Here's how the part is built. I have some questions about the finished solid (model axes, mm). A direction names the side the tool comes from. Round coordinates to 2 decimals unless told otherwise and drop trailing zeros. Loops run counter-clockwise (first coordinate to the right, second up) from the corner with the lowest first, then second, coordinate; pieces in that order, holes last. Notation, with made-up numbers: (-21.75, 0.25) - (8.25, 0.25) arc R24 cw to (8.25, 12.25) - close; hole circle Ø3 at (-23.5, 72.5). An arc over 180 degrees is marked (long way). Answer as a JSON object with one key per item and string values. Group by question number.
1) I want a section at A-A, the plane x = -8.05. Please give me the cut outline in (y, z), then the cut area to 3 significant figures.
2) If I drill on line 1 along Y through (x, z) = (0, 17.95); line 2 along Z through (x, y) = (14, 29); line 3 along X through (y, z) = (28, 18.5), over which ranges is the centre line in solid material (lowest first)? Write a range as [from, to].
3) I want a section at C-C, the plane z = 8.05. Please give me the cut outline in (x, y), then the cut area to 3 significant figures.
4) Which directions (+Z, -Z, +X, -X, +Y, -Y) give clear straight access to the entire face, cutting with the end or side of a thin tool? Please do faces 1 (the face through (0, 26, -17)), 2 (the face through (0.08, 26.25, -18.48)).
5) I want a section at B-B, the plane y = 28.05. Please give me the cut outline in (x, z), then the cut area to 3 significant figures.
6) I want a section at D-D, the plane x = 14. Please give me the cut outline in (y, z), then the cut area to 3 significant figures.
7) If we mould it in two halves opening along Y, with no side actions, what happens to faces 3 (the face through (0, 40, -19)), 4 (the face through (-7.45, 1.52, 5.3)), 5 (the face through (-6.265, 20.234, 18.479))? For each: pulls with the +Y half, pulls with the -Y half, needs draft (parallel to the pull), parting line crosses it, or undercut.
8) Will these pins go through, and if not, where does the flat tip stop? P1, Ø10, axis at x = 9, z = 5.5, coming from the +Y side; P2, Ø3, axis at x = -5.69, z = 5.69, coming from the +Y side.
from build123d import *

# Parameters (mm, degrees)
C_1U_DEPTH               = 20
SKETCH_8_R               = 3.95
SKETCH_8_R_2             = 1.8
CUT_EXTRUDE_696_DEPTH    = 5
PATTERN_CIRCULAR_A_COUNT = 2
PATTERN_CIRCULAR_A_ANGLE = 270
PATTERN_CIRCULAR_B_COUNT = 2
PATTERN_CIRCULAR_B_ANGLE = 90


with BuildPart() as part:
    # c型梁 → C型梁1u (new, symmetric)
    with BuildSketch(Plane(origin=(0, 0, 0), x_dir=(0, 0, -1), z_dir=(1, 0, 0))):
        Polygon((-20, 0), (20, 0), (20, 40), (17, 40), (17, 3), (-17, 3), (-17, 40), (-20, 40), align=None)
    extrude(amount=C_1U_DEPTH, both=True)

    # 8位安装孔 → Cut-Extrude 696 (cut, symmetric)
    with BuildSketch(Plane(origin=(0, 3, 0), x_dir=(1, 0, 0), z_dir=(0, 1, 0))):
        with Locations(Location((0, 0, 0), (0, 0, 270))):
            Circle(SKETCH_8_R)
        with Locations(Location((8.05, 0, 0), (0, 0, 270))):
            Circle(SKETCH_8_R_2)
        with Locations(Location((5.692209589, -5.692209589, 0), (0, 0, 270))):
            Circle(SKETCH_8_R_2)
        with Locations(Location((0, -8.05, 0), (0, 0, 270))):
            Circle(SKETCH_8_R_2)
        with Locations(Location((-5.692209589, -5.692209589, 0), (0, 0, 270))):
            Circle(SKETCH_8_R_2)
        with Locations(Location((-8.05, 0, 0), (0, 0, 270))):
            Circle(SKETCH_8_R_2)
        with Locations(Location((-5.692209589, 5.692209589, 0), (0, 0, 270))):
            Circle(SKETCH_8_R_2)
        with Locations(Location((0, 8.05, 0), (0, 0, 270))):
            Circle(SKETCH_8_R_2)
        with Locations(Location((5.692209589, 5.692209589, 0), (0, 0, 270))):
            Circle(SKETCH_8_R_2)
    cut_extrude_696 = extrude(amount=CUT_EXTRUDE_696_DEPTH, both=True, mode=Mode.SUBTRACT)

    # 安装孔A侧: Cut-Extrude 696 ×2 about axis
    pattern_circular_a_axis = Axis((20, 3, 17), (-1, 0, 0))
    for i in range(1, PATTERN_CIRCULAR_A_COUNT):
        add(cut_extrude_696.rotate(pattern_circular_a_axis, i * PATTERN_CIRCULAR_A_ANGLE / (PATTERN_CIRCULAR_A_COUNT - 1)), mode=Mode.SUBTRACT)

    # 安装孔B侧: Cut-Extrude 696 ×2 about axis
    pattern_circular_b_axis = Axis((20, 3, -17), (-1, 0, 0))
    for i in range(1, PATTERN_CIRCULAR_B_COUNT):
        add(cut_extrude_696.rotate(pattern_circular_b_axis, i * PATTERN_CIRCULAR_B_ANGLE / (PATTERN_CIRCULAR_B_COUNT - 1)), mode=Mode.SUBTRACT)


solid = part.part
Outcome:
{
 "1": {"outline": "(0, -20) - (18.2, -20) - (18.2, -17) - (3, -17) - (3, -1.8) - (0, -1.8) - close; (0, 1.8) - (3, 1.8) - (3, 17) - (18.2, 17) - (18.2, 20) - (0, 20) - close; (21.8, -20) - (40, -20) - (40, -17) - (21.8, -17) - close; (21.8, 17) - (40, 17) - (40, 20) - (21.8, 20) - close", "area": "310 mm^2"},
 "2": {"line 1": "[0, 10.15], [13.75, 16.05], [23.95, 26.25], [29.85, 40]", "line 2": "[-20, -17], [17, 20]", "line 3": "[-20, -1.8], [1.8, 20]"},
 "3": {"outline": "(-20, 0) - (-1.8, 0) - (-1.8, 3) - (-20, 3) - close; (1.8, 0) - (20, 0) - (20, 3) - (1.8, 3) - close", "area": "109 mm^2"},
 "4": {"face 1": "+X, -X, +Y", "face 2": "+Z, -Z"},
 "5": {"outline": "(-20, -20) - (-1.8, -20) - (-1.8, -17) - (-20, -17) - close; (-20, 17) - (-1.8, 17) - (-1.8, 20) - (-20, 20) - close; (1.8, -20) - (20, -20) - (20, -17) - (1.8, -17) - close; (1.8, 17) - (20, 17) - (20, 20) - (1.8, 20) - close", "area": "218 mm^2"},
 "6": {"outline": "(0, -20) - (40, -20) - (40, -17) - (3, -17) - (3, 17) - (40, 17) - (40, 20) - (0, 20) - close", "area": "342 mm^2"},
 "7": {"face 3": "pulls with the +Y half", "face 4": "needs draft", "face 5": "undercut"},
 "8": {"P1": "y = 3", "P2": "through"}
}
